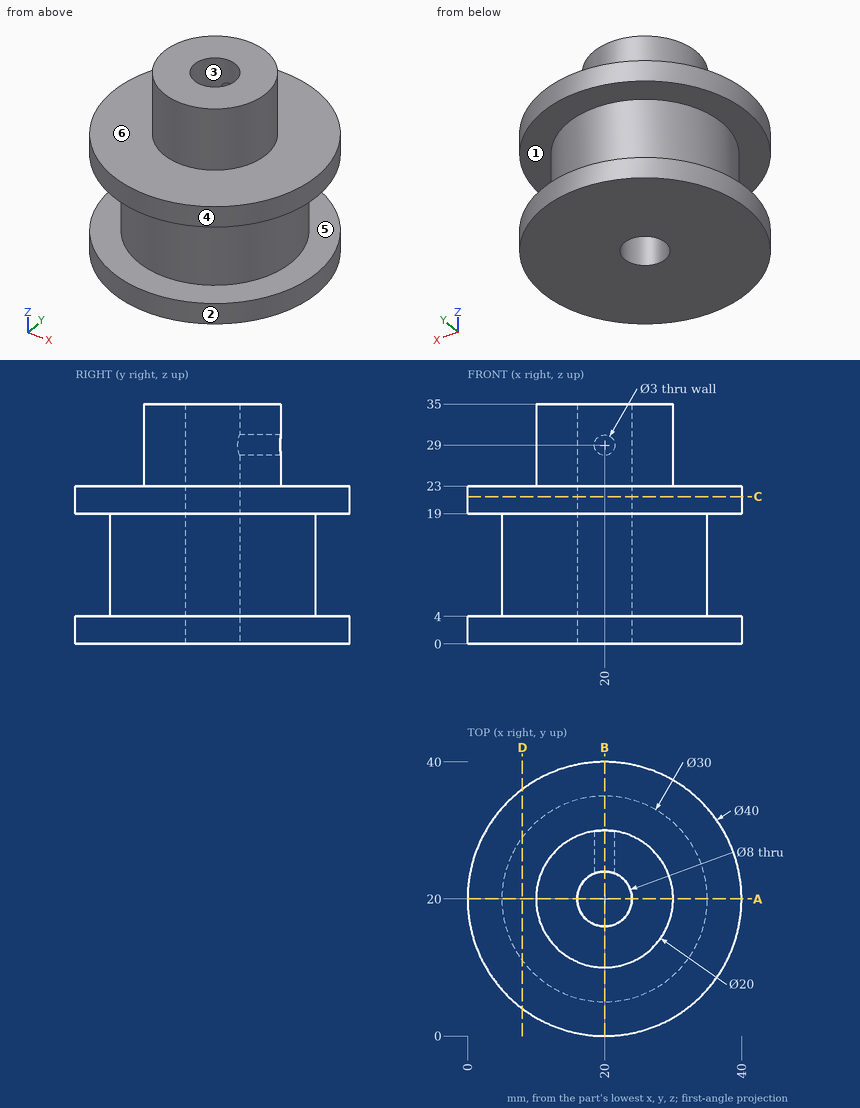
Part print with two shaded views. Sizes in mm from the minimum x, y, z corner. A direction names the side the tool comes from. Coordinates: 2 decimals unless noted, no trailing zeros. Write each loop counter-clockwise with the first axis right and the second up, starting at its lowest first coordinate (ties: lowest second). Pieces come first, ordered by that corner, then holes.
1. 3-axis set-ups, long thin cutter, end or side, ignore diameter. For the marked faces 4, 5 and 6: which of +Z, -Z, +X, -X, +Y, -Y reach the whole face in a straight line?
Answer block:
face 4: +Z, -Z
face 5: none
face 6: +Z
2. Band-saw the part on A-A, the plane y = 20. Give the cut face in (x, z).
Answer block:
outline: (0, 0) - (16, 0) - (16, 35) - (10, 35) - (10, 23) - (0, 23) - (0, 19) - (5, 19) - (5, 4) - (0, 4) - close; (24, 0) - (40, 0) - (40, 4) - (35, 4) - (35, 19) - (40, 19) - (40, 23) - (30, 23) - (30, 35) - (24, 35) - close
3. Band-saw the part on B-B, the plane x = 20. Give the cut face in (y, z), and give its area (3 significant figures).
Answer block:
outline: (0, 0) - (16, 0) - (16, 35) - (10, 35) - (10, 23) - (0, 23) - (0, 19) - (5, 19) - (5, 4) - (0, 4) - close; (24, 0) - (40, 0) - (40, 4) - (35, 4) - (35, 19) - (40, 19) - (40, 23) - (30, 23) - (30, 27.5) - (24, 27.5) - close; (24, 30.5) - (30, 30.5) - (30, 35) - (24, 35) - close
area: 712 mm2
4. Band-saw the part on C-C, the plane z = 21.5. Give the cut face in (x, y).
Answer block:
outline: circle Ø40 at (20, 20); hole circle Ø8 at (20, 20)
5. Pull direction Y, two halves, no side cores. Call the marked faces 1, 2 and 3: released by +Y, released by -Y, zero draft, split by the parting line, or undercut.
Answer block:
face 1: zero draft
face 2: split by the parting line
face 3: undercut
6. Drill centre lines: probe 1 along Z at (x, y) = (2.5, 26); probe 2 along Z at (x, y) = (20, 25.5); probe 3 along Y at (x, z) = (20, 20.5). Where is each one in solid material? Low to high.
Answer block:
probe 1: z = 0 to 4, 19 to 23
probe 2: z = 0 to 27.5, 30.5 to 35
probe 3: y = 0 to 16, 24 to 40
7. Drop flat-ended pins along their axis: pin 1 (2 mm diameter, centred on y = 22, z = 15.5, fed in from +X); pin 2 (1.5 mm diameter, centred on y = 11, z = 17, fed in from -X); pin 3 (1.8 mm diameter, centred on x = 20, z = 29, fed in from -Y). Give the stop position or say it passes through.
Answer block:
pin 1: stops at x = 34.97
pin 2: stops at x = 7.47
pin 3: stops at y = 10
8. Band-saw the part on D-D, the plane x = 8. Give the cut face in (y, z).
Answer block:
outline: (4, 0) - (36, 0) - (36, 4) - (29, 4) - (29, 19) - (36, 19) - (36, 23) - (4, 23) - (4, 19) - (11, 19) - (11, 4) - (4, 4) - close
